The model under review builds one solid part; all positions refer to its coordinate system, in mm. A direction names the side the tool comes from. Coordinates: 2 decimals unless noted, no trailing zeros. Write each loop counter-clockwise with the first axis right and the second up, starting at its lowest first coordinate (ties: lowest second). Pieces come first, ordered by that corner, then holes. Notation, with made-up numbers: (54.5, 80) - (109.5, 80) arc R20 ccw to (109.5, 99) - close; hole circle Ø10 at (-37, 15). An arc over 180 degrees is marked (long way). Put each result on its own line as item: value.
from build123d import *

# Parameters (mm, degrees)
EXTRUDE_1_DEPTH          = 8
CUT_EXTRUDE_1_DEPTH      = 34.079449814
CUT_EXTRUDE_1_DEPTH_BACK = 34.079449814
SKETCH_2_R               = 1.6
SKETCH_2_R_2             = 2.1


with BuildPart() as part:
    # 草图1 → 凸台-拉伸1 (new body)
    with BuildSketch(Plane.XY):
        Polygon((0, 0), (0, 3), (14.5, 3), (14.5, 13), (30.5, 13), (30.5, 0), (26.5, 0), (26.5, 10), (17.5, 10), (17.5, 0), align=None)
    extrude(amount=EXTRUDE_1_DEPTH)

    # 草图2 → 切除-拉伸1 (cut, two sides: drawn at the far end of the back side and taken through both)
    with BuildSketch(Plane.XZ.offset(-10).offset(-CUT_EXTRUDE_1_DEPTH_BACK)):
        with Locations((3, 4)):
            Circle(SKETCH_2_R)
        with Locations((11, 4)):
            Circle(SKETCH_2_R)
        with Locations((22, 4)):
            Circle(SKETCH_2_R_2)
    extrude(amount=CUT_EXTRUDE_1_DEPTH + CUT_EXTRUDE_1_DEPTH_BACK, mode=Mode.SUBTRACT)


solid = part.part
1. Consider section A-A on z = 4. State the section outline as (x, y) points, plus the area to 3 significant figures.
Determined:
outline: (0, 0) - (1.4, 0) - (1.4, 3) - (0, 3) - close; (4.6, 0) - (9.4, 0) - (9.4, 3) - (4.6, 3) - close; (12.6, 0) - (17.5, 0) - (17.5, 10) - (19.9, 10) - (19.9, 13) - (14.5, 13) - (14.5, 3) - (12.6, 3) - close; (24.1, 10) - (26.5, 10) - (26.5, 0) - (30.5, 0) - (30.5, 13) - (24.1, 13) - close
area: 130 mm^2
2. For pin 1 Ø4 at (x, z) = (3, 4) entering from +Y; pin 2 Ø2.5 at (y, z) = (6, 4.5) entering from -X, all flat-tipped, find the tip position at first contact; note any pin that passes through.
Determined:
pin 1: stops at y = 3
pin 2: stops at x = 14.5
3. Consider section B-B on x = 3. State the section outline as (y, z) points, plus the area to 3 significant figures.
Determined:
outline: (0, 0) - (3, 0) - (3, 2.4) - (0, 2.4) - close; (0, 5.6) - (3, 5.6) - (3, 8) - (0, 8) - close
area: 14.4 mm^2
4. The part is to be moulded in two halves that separate along X. For faces 1 (the flat face through (14.5, 8, 4)), 2 (the flat face through (24.1, 10, 3.1)), 3 (the flat face through (24.2, 13, 4.8)), 4 (the flat face through (26.5, 5, 4)), say which applies: +X half, -X half, draft (parallel to the pull), parting line (faces both ways), or undercut.
Determined:
face 1: -X half
face 2: undercut
face 3: draft
face 4: undercut
5. Machinability: for faces 5 (the flat face through (17.5, 5, 4)), 6 (the flat face through (29, 0, 4)), 7 (the flat face through (7, 3, 4)), which of the approach directions +Z, -Z, +X, -X, +Y, -Y give a long, thin tool a straight path to every point of the face, cutting with its end or side? Answer none if there is none.
Determined:
face 5: +Z, -Z, -Y
face 6: +Z, -Z, +X, -X, -Y
face 7: +Z, -Z, -X, +Y
6. Consider section C-C on y = 7.5. State the section outline as (x, z) points.
Determined:
outline: (14.5, 0) - (17.5, 0) - (17.5, 8) - (14.5, 8) - close; (26.5, 0) - (30.5, 0) - (30.5, 8) - (26.5, 8) - close
7. Consider section D-D on z = 1.25. State the section outline as (x, y) points.
Determined:
outline: (0, 0) - (17.5, 0) - (17.5, 10) - (26.5, 10) - (26.5, 0) - (30.5, 0) - (30.5, 13) - (14.5, 13) - (14.5, 3) - (0, 3) - close
8. To check wall thickness, follow probe 1 along X at (y, z) = (1.3, 4); probe 2 along X at (y, z) = (11.7, 4); probe 3 along Z at (x, y) = (3, 1.9). State the ranges of each line that lie inside material, in increasing order.
Determined:
probe 1: x = 0 to 1.4, 4.6 to 9.4, 12.6 to 17.5, 26.5 to 30.5
probe 2: x = 14.5 to 19.9, 24.1 to 30.5
probe 3: z = 0 to 2.4, 5.6 to 8
